Geometry check sheet. Reference: drawing and pictorial views, mm from the part's lowest x, y, z. Coordinates: 2 decimals unless noted, no trailing zeros. Loops run counter-clockwise (first coordinate to the right, second up) from the corner with the lowest first, then second, coordinate; pieces in that order, holes last. Notation, with made-up numbers: (20.5, 28.25) - (65.5, 28.25) arc R14 ccw to (65.5, 51.25) - close; hole circle Ø10 at (-18.75, 78.25). An arc over 180 degrees is marked (long way). Write each question's results on one line, items separated by ' | '. Start each with the question number.
1. Cross-section at A-A (y = 13.5). Record the cut outline in (x, z).
2. Cross-section at D-D (x = 22.5). Record the cut outline in (y, z) (3 decimals).
3. Thickness scan on line 1 (Y direction, x = 2, z = 110); line 2 (X direction, y = 16.75, z = 91); line 3 (Y direction, x = 35, z = 20) (3 decimals). Record the ranges inside material, lowest first. Write a range as [from, to].
4. Cross-section at C-C (z = 130). Record the cut outline in (x, y) (3 decimals), and give its area (3 significant figures).
5. Cross-section at B-B (z = 110). Record the cut outline in (x, y) (3 decimals), and give its area (3 significant figures).
6. Draft check along X on the marked faces 1, 2, 3 and 4. Enter one of: released by +X, released by -X, zero draft, split by the parting line, or undercut.
7. Gauge pin test, flat ends, axial feed: P1, Ø3, axis at x = 23.5, z = 113.5, coming from the +Y side (3 decimals); P2, Ø4.5, axis at y = 13.5, z = 110, coming from the +X side. Record the tip position at first contact, or that the pin passes through.
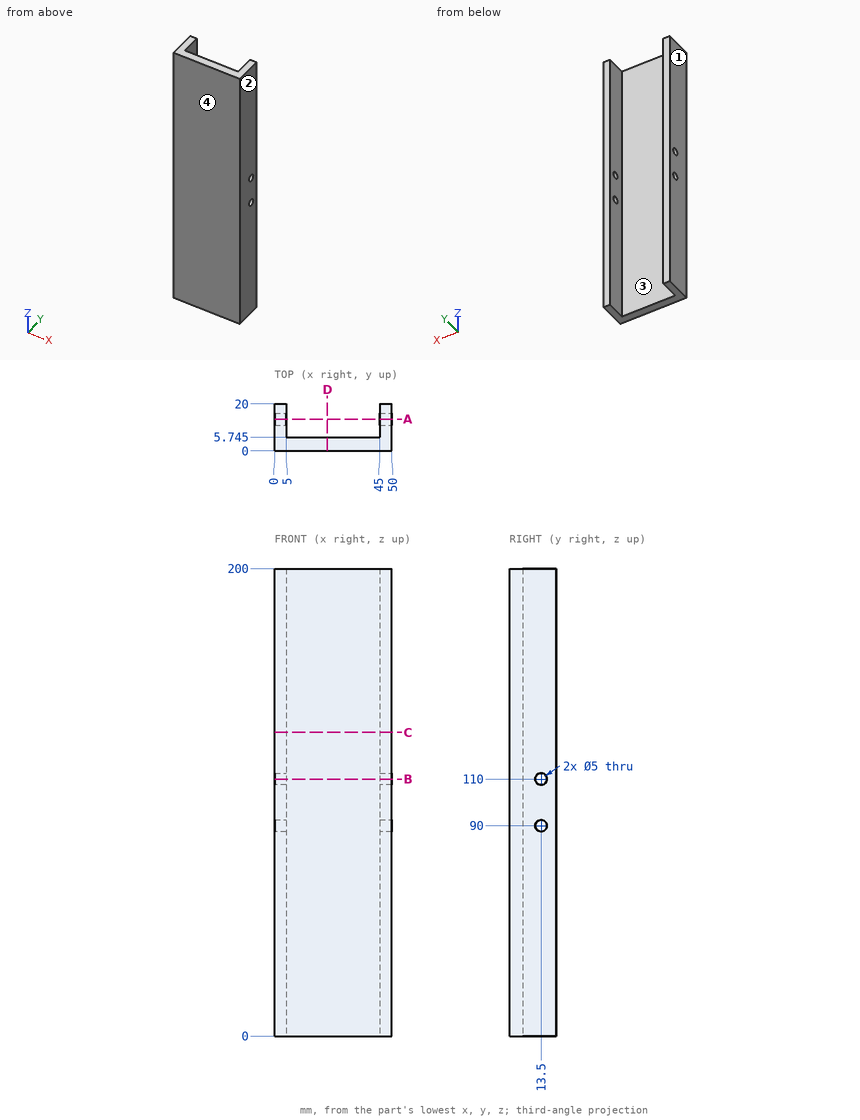
Established:
1) outline: (0, 0) - (5, 0) - (5, 87.5) - (0, 87.5) - close; (0, 92.5) - (5, 92.5) - (5, 107.5) - (0, 107.5) - close; (0, 112.5) - (5, 112.5) - (5, 200) - (0, 200) - close; (45, 0) - (50, 0) - (50, 87.5) - (45, 87.5) - close; (45, 92.5) - (50, 92.5) - (50, 107.5) - (45, 107.5) - close; (45, 112.5) - (50, 112.5) - (50, 200) - (45, 200) - close
2) outline: (0, 0) - (5.745, 0) - (5.745, 200) - (0, 200) - close
3) line 1: [0, 11], [16, 20] | line 2: [0, 5], [45, 50] | line 3: [0, 5.745]
4) outline: (0, 0) - (50, 0) - (50, 20) - (45, 20) - (45, 5.745) - (5, 5.745) - (5, 20) - (0, 20) - close | area: 430 mm^2
5) outline: (0, 0) - (50, 0) - (50, 11) - (45, 11) - (45, 5.745) - (5, 5.745) - (5, 11) - (0, 11) - close; (0, 16) - (5, 16) - (5, 20) - (0, 20) - close; (45, 16) - (50, 16) - (50, 20) - (45, 20) - close | area: 380 mm^2
6) face 1: released by -X | face 2: released by +X | face 3: undercut | face 4: zero draft
7) P1: y = 5.745 | P2: through
